Check sheet for the drawn part. Datum: minimum x, y, z corner. Units: mm. A direction names the side the tool comes from. Give positions to 0.01 mm unless a question says otherwise; leave off trailing zeros. Write each loop counter-clockwise with the first axis right and the second up, starting at its lowest first coordinate (ties: lowest second). Pieces come first, ordered by that corner, then holes. Notation, with made-up numbers: M 25.5,40.25 L 31.5,40.25 A19 ccw 31.5,56.25 Z; hole C -34,-3 d7. An arc over 180 degrees is marked long. Use CSV: the item, a comma, the result in double quotes. Start each with the question number.
1. Cross-section at A-A, the plane y = 12.5. Enter the section's corners in (x, z), and give its area (3 significant figures).
2. Mould release check, pull along Y, two halves, no side actions. Record for the marked faces 3, 4, 5 and 6: +Y half, -Y half, draft (parallel to the pull), parting line (faces both ways), or undercut.
3. Depth check by flat-ended pin: P1, Ø1, axis at x = 17.5, y = 21.5, coming from the -Z side; P2, Ø2, axis at y = 13.5, z = 25.5, coming from the +X side; P3, Ø4, axis at x = 20, z = 7.5, coming from the +Y side; P4, Ø3, axis at y = 10.5, z = 26.5, coming from the -X side. Enter the tip coordinate at first touch or a pass-through.
4. Cross-section at D-D, the plane z = 13. Enter the section's corners in (x, y), and give its area (3 significant figures).
5. Access from +Z, -Z, +X, -X, +Y, -Y to the whole of each face (thin tool, end or side, straight path). Record for the marked faces 1 and 2.
6. Scan lines: line 1 (Y direction, x = 12.5, z = 16); line 2 (Z direction, x = 18.25, y = 18); line 3 (Y direction, x = 12, z = 4.5). Record each from-to range of solid material in increasing order.
7. Cross-section at C-C, the plane x = 8. Enter the section's corners in (y, z), and give its area (3 significant figures).
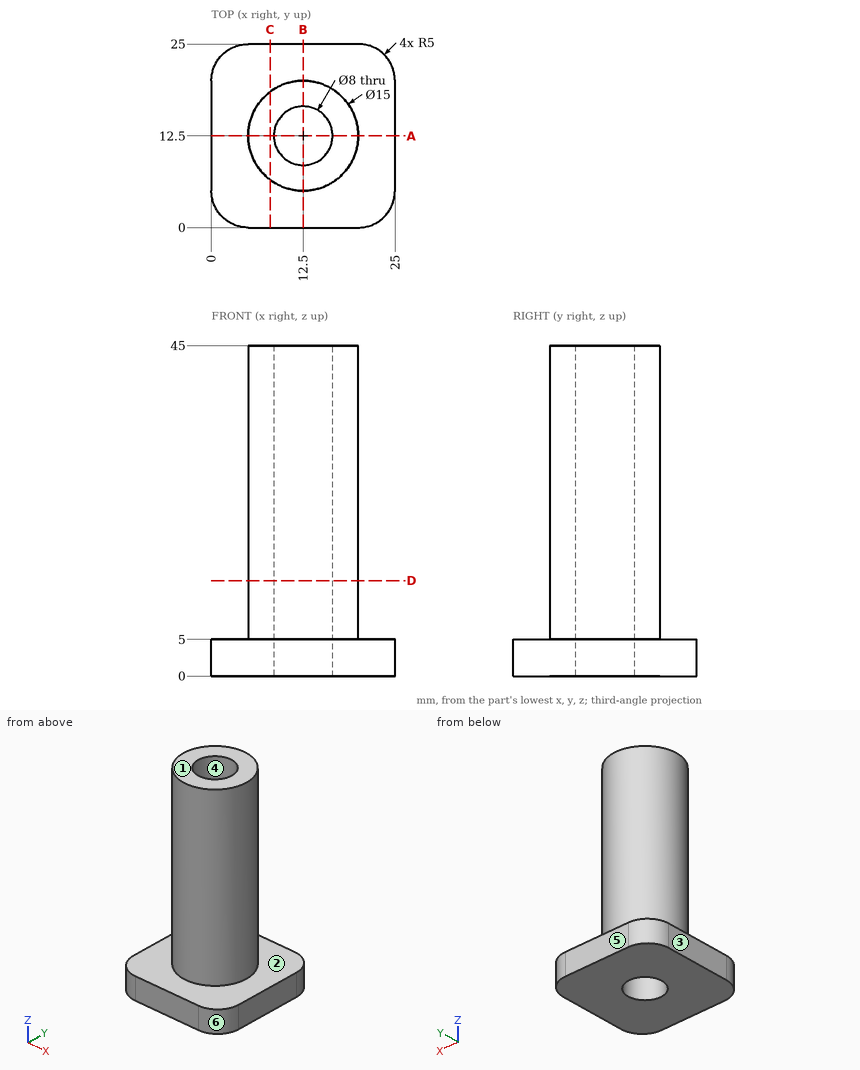
Worked answers:
1,outline,"M 0,0 L 8.5,0 L 8.5,45 L 5,45 L 5,5 L 0,5 Z; M 16.5,0 L 25,0 L 25,5 L 20,5 L 20,45 L 16.5,45 Z"
1,area,"365 mm^2"
2,face 3,"draft"
2,face 4,"undercut"
2,face 5,"+Y half"
2,face 6,"-Y half"
3,P1,"stops at z = 0"
3,P2,"stops at x = 20"
3,P3,"stops at y = 17.6"
3,P4,"stops at x = 5.02"
4,outline,"C 12.5,12.5 d15; hole C 12.5,12.5 d8"
4,area,"126 mm^2"
5,face 1,"+Z, +X, -X, +Y, -Y"
5,face 2,"+Z"
6,line 1,"y = 5 to 8.5, 16.5 to 20"
6,line 2,"z = 0 to 5"
6,line 3,"y = 0 to 8.53, 16.47 to 25"
7,outline,"M 0,0 L 25,0 L 25,5 L 18.5,5 L 18.5,45 L 6.5,45 L 6.5,5 L 0,5 Z"
7,area,"605 mm^2"
